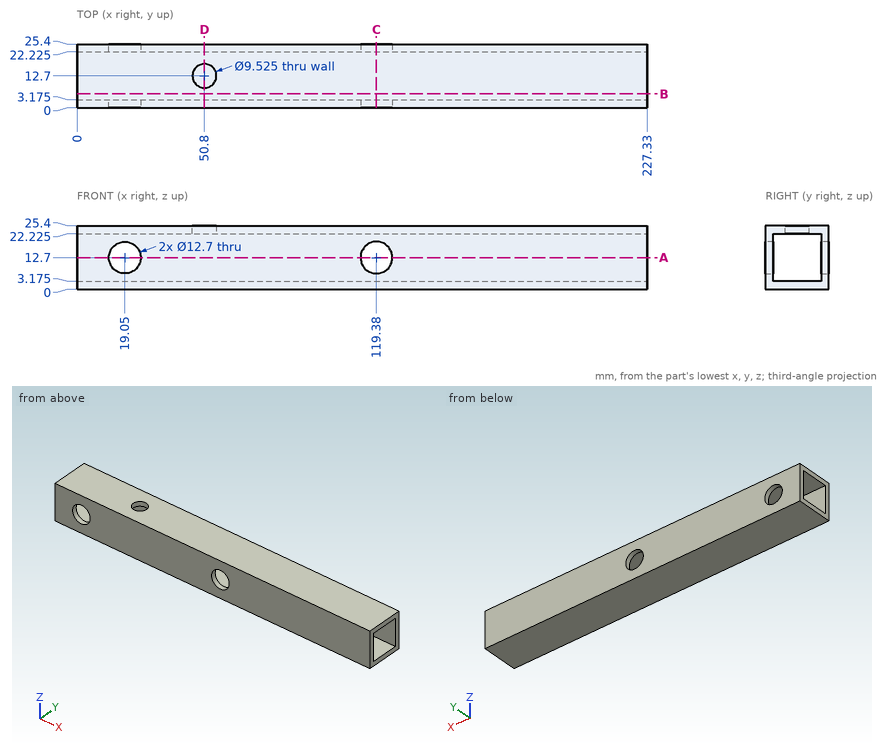
Part print with two shaded views. Sizes in mm from the minimum x, y, z corner. Coordinates: 2 decimals unless noted, no trailing zeros. Loops run counter-clockwise (first coordinate to the right, second up) from the corner with the lowest first, then second, coordinate; pieces in that order, holes last. Notation, with made-up numbers: M -17.75,-25 L 34.25,-25 A24 cw 34.25,4 Z; hole C 63,-24 d8. An arc over 180 degrees is marked long. Use CSV: the item, a comma, the result in double quotes. Start each with the question number.
1. Band-saw the part on D-D, the plane x = 50.8. List the corners of the cut face in (y, z) (1 decimal).
2. Flat gauge pin, fed straight in: pin 1 (10 mm diameter, centred on x = 19.05, z = 12.7, fed in from -Y). Where does the tip first touch, or does it go through?
3. Band-saw the part on C-C, the plane x = 119.38. List the corners of the cut face in (y, z) (3 decimals).
4. Band-saw the part on B-B, the plane y = 5.5. List the corners of the cut face in (x, z) (3 decimals), then the cut area to 3 significant figures.
5. Band-saw the part on A-A, the plane z = 12.7. List the corners of the cut face in (x, y) (3 decimals).
6. Probe probe 1 along X at (y, z) = (1.35, 12.7); probe 2 along Y at (x, z) = (44.5, 9.75) (3 decimals). List the from-to ranges inside material, lowest first. Write a range as [from, to].
Entries:
1,outline,"M 0,0 L 25.4,0 L 25.4,25.4 L 17.5,25.4 L 17.5,22.2 L 22.2,22.2 L 22.2,3.2 L 3.2,3.2 L 3.2,22.2 L 7.9,22.2 L 7.9,25.4 L 0,25.4 Z"
2,pin 1,"passes through"
3,outline,"M 0,0 L 25.4,0 L 25.4,6.35 L 22.225,6.35 L 22.225,3.175 L 3.175,3.175 L 3.175,6.35 L 0,6.35 Z; M 0,19.05 L 3.175,19.05 L 3.175,22.225 L 22.225,22.225 L 22.225,19.05 L 25.4,19.05 L 25.4,25.4 L 0,25.4 Z"
4,outline,"M 0,0 L 227.33,0 L 227.33,3.175 L 0,3.175 Z; M 0,22.225 L 227.33,22.225 L 227.33,25.4 L 0,25.4 Z"
4,area,"1,440 mm2"
5,outline,"M 0,0 L 12.7,0 L 12.7,3.175 L 0,3.175 Z; M 0,22.225 L 12.7,22.225 L 12.7,25.4 L 0,25.4 Z; M 25.4,0 L 113.03,0 L 113.03,3.175 L 25.4,3.175 Z; M 25.4,22.225 L 113.03,22.225 L 113.03,25.4 L 25.4,25.4 Z; M 125.73,0 L 227.33,0 L 227.33,3.175 L 125.73,3.175 Z; M 125.73,22.225 L 227.33,22.225 L 227.33,25.4 L 125.73,25.4 Z"
6,probe 1,"x = [0, 12.7], [25.4, 113.03], [125.73, 227.33]"
6,probe 2,"y = [0, 3.175], [22.225, 25.4]"
